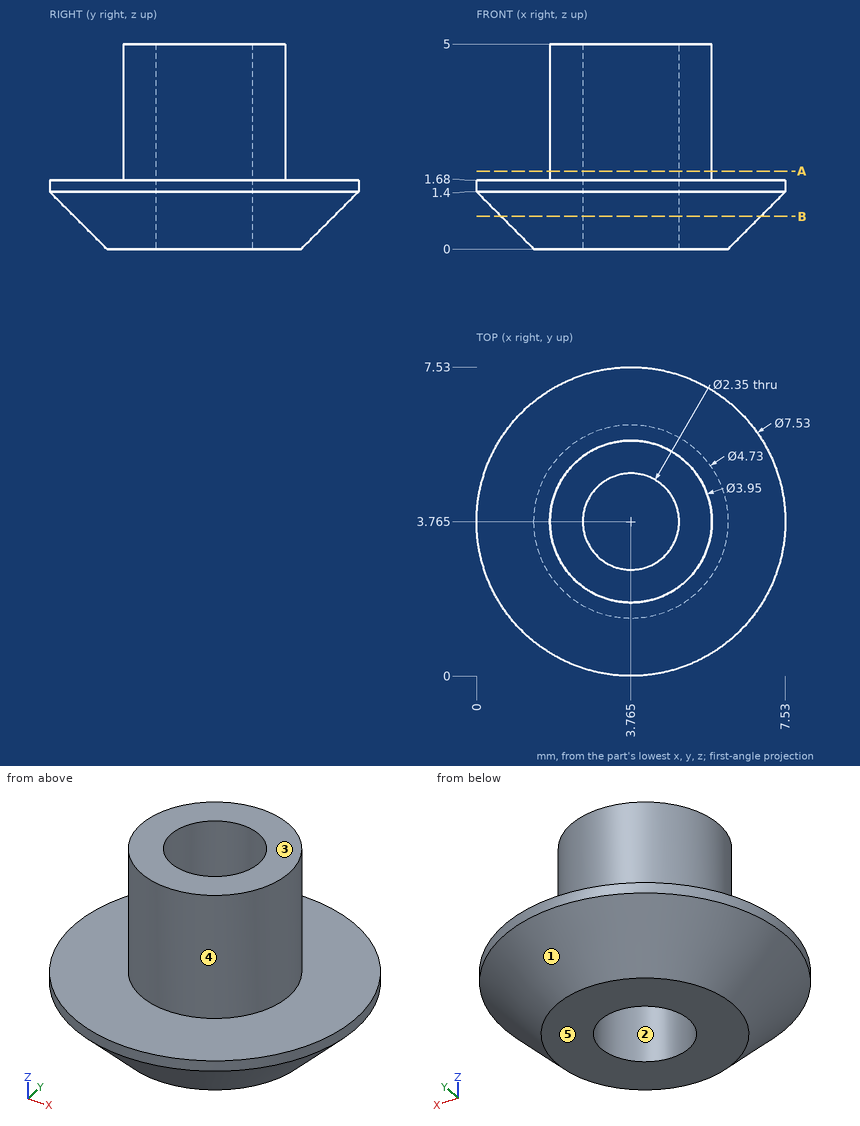
The figure shows three views and two pictorial views of one solid part (mm, origin at its lowest corner). Answer the questions. A direction names the side the tool comes from. Round coordinates to 2 decimals unless told otherwise and drop trailing zeros. Order: outer loops, then holes, each group sorted by start corner. A loop starts at its lowest first (then second) coordinate and runs counter-clockwise, first axis right, second up.
Q1. A cutting plane is placed at A-A, the plane z = 1.9. Determine the outline of the cut face in (x, y) (3 decimals).
Solution:
outline: circle Ø3.95 at (3.765, 3.765); hole circle Ø2.35 at (3.765, 3.765)
Q2. A tool of negligible diameter and unlimited length cuts with its end or side. For the marked faces 4 and 5, from which of +Z, -Z, +X, -X, +Y, -Y can it reach the whole face along a straight path? Write none if from no direction.
Solution:
face 4: +Z
face 5: -Z, +X, -X, +Y, -Y
Q3. The mould has two halves that part along X. Classify the marked faces 1, 2 and 3: pulls with the +X half, pulls with the -X half, needs draft (parallel to the pull), parting line crosses it, or undercut.
Solution:
face 1: parting line crosses it
face 2: undercut
face 3: needs draft
Q4. A cutting plane is placed at B-B, the plane z = 0.8. Determine the outline of the cut face in (x, y) (3 decimals).
Solution:
outline: circle Ø6.33 at (3.765, 3.765); hole circle Ø2.35 at (3.765, 3.765)
Q5. Find the intervals of material crossed by line 1 along Z through (x, y) = (4.5, 5.75); line 2 along Y through (x, z) = (3, 1.8); line 3 along Y through (x, z) = (4, 2.65), in increasing order.
Solution:
line 1: z = 0 to 1.68
line 2: y = 1.94 to 2.87, 4.66 to 5.59
line 3: y = 1.8 to 2.61, 4.92 to 5.73
Q6. Given pin 1 Ø2 at (y, z) = (1, 3) entering from +X; pin 2 Ø1.5 at (x, z) = (1.5, 4) entering from -Y, each flat-ended and moving along its own axis, determine where each tip first touches the part or whether it passes through.
Solution:
pin 1: stops at x = 4.65
pin 2: stops at y = 2.5
